Can you work these out from the model? Positions are in its coordinate system, mm. A direction names the side the tool comes from. Round coordinates to 2 decimals unless told otherwise and drop trailing zeros. Write each loop counter-clockwise with the first axis right and the second up, starting at its lowest first coordinate (ties: lowest second). Pieces come first, ordered by that corner, then holes. Notation, with made-up numbers: M 27,10 L 50,10 A16 ccw 50,28 Z; hole C 80.25,11 d6. An arc over 180 degrees is marked long. Answer in a Markdown table with one row per item. Add a question column.
(1) If we mould it in two halves opening along Y, with no side actions, what happens to faces 1 (the face through (-2, 28, 3)), 2 (the face through (-20, 0, 7)), 3 (the face through (-13.834, 9.633, 7.395)), 4 (the face through (-3, 10, 7))? For each: released by +Y, released by -Y, zero draft, split by the parting line, or undercut.
(2) Suppose I cut it at D-D, the plane y = 10. Write out the boundary of the cut face in (x, z), then the cut area to 3 significant figures.
(3) If I drill on probe 1 along X at (y, z) = (28.5, 8.75); probe 2 along X at (y, z) = (7.75, 9.75); probe 3 along X at (y, z) = (6.5, 11), over which ranges is the centre line in solid material (lowest first)?
(4) Suppose I cut it at A-A, the plane z = 14. Write out the boundary of the cut face in (x, y).
(5) Suppose I cut it at B-B, the plane x = -11. Write out the boundary of the cut face in (y, z), then the cut area to 3 significant figures.
(6) Suppose I cut it at C-C, the plane y = 2. Write out the boundary of the cut face in (x, z), then the cut area to 3 significant figures.
(7) For faces 5 (the face through (-3, 24, 7)), 6 (the face through (-14, 3, 7)), 7 (the face through (-37, 1, 13)), which set-ups out of +Z, -Z, +X, -X, +Y, -Y let a thin tool reach every point of the face, with its end or its side?
(8) I'm going to push flat-ended pins straight in: pin 1 (3 mm diameter, centred on x = -36, z = 5, fed in from +Y); pin 2 (4.5 mm diameter, centred on x = -14, z = 8, fed in from +Y); pin 3 (2 mm diameter, centred on y = 25.5, z = 3, fed in from -X). Where does each tip first touch, or does it pass through?
from build123d import *

# Parameters (mm, degrees)
PAD_DEPTH       = 15
CHAMFER_SIZE    = 5
CHAMFER001_SIZE = 5


with BuildPart() as part:
    # Sketch → Pad (new body)
    with BuildSketch(Plane.XY):
        Polygon((0, 0), (-40, 0), (-40, 3), (-30, 3), (-3, 20), (-3, 30), (0, 30), align=None)
        Polygon((-3, 3), (-24.36951, 3), (-3, 16.454876), align=None, mode=Mode.SUBTRACT)
    extrude(amount=PAD_DEPTH)

    # Chamfer
    chamfer_edges = [part.edges().sort_by_distance(p)[0] for p in [
        (-40, 1.5, 0),
        (-40, 1.5, 15),
    ]]
    chamfer(chamfer_edges, length=CHAMFER_SIZE)

    # Chamfer001
    chamfer001_edges = [part.edges().sort_by_distance(p)[0] for p in [
        (-1.5, 30, 0),
        (-1.5, 30, 15),
    ]]
    chamfer(chamfer001_edges, length=CHAMFER001_SIZE)


solid = part.part
Calculated:
| question | item | result |
|---|---|---|
| 1 | face 1 | released by +Y |
| 1 | face 2 | released by -Y |
| 1 | face 3 | undercut |
| 1 | face 4 | undercut |
| 2 | outline | M -18.88,0 L -13.25,0 L -13.25,15 L -18.88,15 Z; M -3,0 L 0,0 L 0,15 L -3,15 Z |
| 2 | area | 129 mm² |
| 3 | probe 1 | -3 to 0 |
| 3 | probe 2 | -22.46 to -16.83, -3 to 0 |
| 3 | probe 3 | -24.44 to -18.81, -3 to 0 |
| 4 | outline | M -36,0 L 0,0 L 0,26 L -3,26 L -3,20 L -30,3 L -36,3 Z; hole M -24.37,3 L -3,3 L -3,16.45 Z |
| 5 | outline | M 0,0 L 3,0 L 3,15 L 0,15 Z; M 11.42,0 L 14.96,0 L 14.96,15 L 11.42,15 Z |
| 5 | area | 98.2 mm² |
| 6 | outline | M -40,5 L -35,0 L 0,0 L 0,15 L -35,15 L -40,10 Z |
| 6 | area | 575 mm² |
| 7 | face 5 | +Z, -Z, -X, +Y |
| 7 | face 6 | +Z, -Z |
| 7 | face 7 | +Z, -X, +Y, -Y |
| 8 | pin 1 | y = 3 |
| 8 | pin 2 | y = 14.49 |
| 8 | pin 3 | x = -3 |
